The drawing under review shows one solid part. Ordinate dimensions are in mm from its lowest x, y, z. Round coordinates to 2 decimals unless told otherwise and drop trailing zeros. Loops run counter-clockwise (first coordinate to the right, second up) from the corner with the lowest first, then second, coordinate; pieces in that order, holes last. Notation, with made-up numbers: M 76.5,12.25 L 117.5,12.25 A12 ccw 117.5,35.25 Z; hole C 70,52.25 d9. An arc over 180 degrees is marked long. Use a Markdown table: item, result.
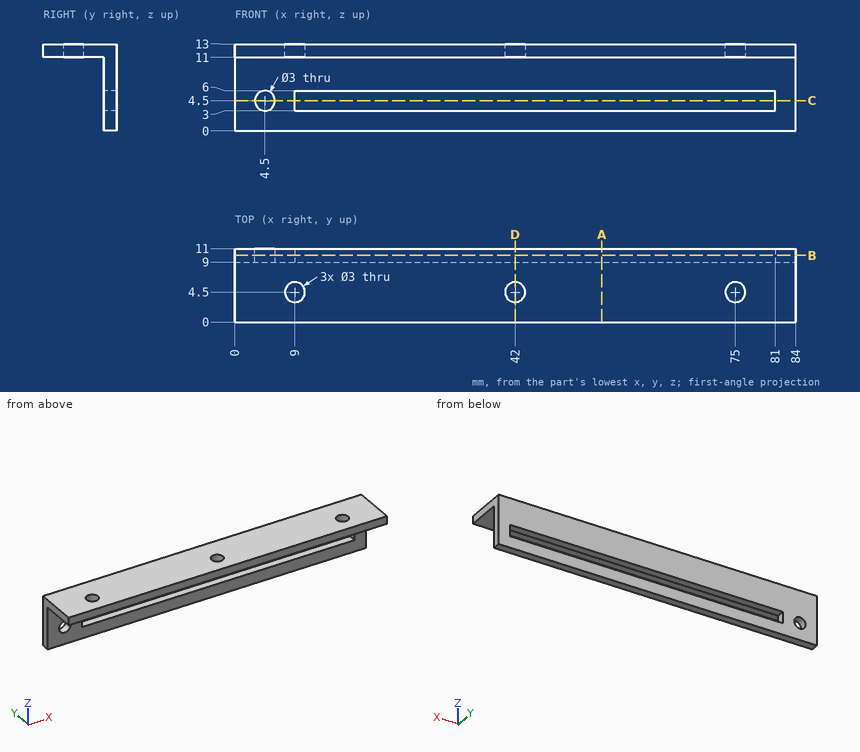
1. Wall thickness on line 1 along Y through (x, z) = (75, 12.1); line 2 along Z through (x, y) = (26, 10.75); line 3 along X through (y, z) = (3.5, 11.25): over which ranges is each line inside the solid? List them lowest first. Write a range as from..to.
Check values:
| item | result |
|---|---|
| line 1 | y = 0..3, 6..11 |
| line 2 | z = 0..3, 6..13 |
| line 3 | x = 0..7.88, 10.12..40.88, 43.12..73.88, 76.12..84 |
2. Take a section at C-C on z = 4.5. Give the boundary of the cut face in (x, y).
Check values:
| item | result |
|---|---|
| outline | M 0,9 L 3,9 L 3,11 L 0,11 Z; M 6,9 L 9,9 L 9,11 L 6,11 Z; M 81,9 L 84,9 L 84,11 L 81,11 Z |
3. Take a section at D-D on x = 42. Give the boundary of the cut face in (y, z).
Check values:
| item | result |
|---|---|
| outline | M 0,11 L 3,11 L 3,13 L 0,13 Z; M 6,11 L 9,11 L 9,6 L 11,6 L 11,13 L 6,13 Z; M 9,0 L 11,0 L 11,3 L 9,3 Z |
4. Take a section at B-B on y = 10. Give the boundary of the cut face in (x, z), and give its area (3 significant figures).
Check values:
| item | result |
|---|---|
| outline | M 0,0 L 84,0 L 84,13 L 0,13 Z; hole C 4.5,4.5 d3; hole M 9,3 L 81,3 L 81,6 L 9,6 Z |
| area | 869 mm² |
5. Take a section at A-A on x = 55. Give the boundary of the cut face in (y, z), and give its area (3 significant figures).
Check values:
| item | result |
|---|---|
| outline | M 0,11 L 9,11 L 9,6 L 11,6 L 11,13 L 0,13 Z; M 9,0 L 11,0 L 11,3 L 9,3 Z |
| area | 38.0 mm² |
6. Insertion check: pin 1 (4.5 mm diameter, centred on x = 43, y = 3, fed in from -Z); pin 2 (5.5 mm diameter, centred on x = 61, z = 4.5, fed in from -Y). Each pin has a flat end and moves straight along its axis. Give the tip position at first contact, or say it passes through.
Check values:
| item | result |
|---|---|
| pin 1 | stops at z = 11 |
| pin 2 | stops at y = 9 |
